```python
from build123d import *

# Parameters (mm, degrees)
SKETCH1_W           = 500
SKETCH1_H           = 775
BOSS_EXTRUDE1_DEPTH = 50
SKETCH2_R           = 8
CUT_EXTRUDE1_DEPTH  = 45
CUT_EXTRUDE2_START  = -45
SKETCH3_R           = 8
CUT_EXTRUDE2_DEPTH  = 45
SKETCH4_R           = 66.548277476
BOSS_EXTRUDE2_DEPTH = 60.75
FILLET1_R           = 60


with BuildPart() as part:
    # Sketch1 → Boss-Extrude1 (new body)
    with BuildSketch(Plane(origin=(0, 0, 0), x_dir=(1, 0, 0), z_dir=(0, 1, 0))):
        with Locations((250, 387.5)):
            Rectangle(SKETCH1_W, SKETCH1_H)
    extrude(amount=BOSS_EXTRUDE1_DEPTH)

    # Sketch2 → Cut-Extrude1 (cut)
    with BuildSketch(Plane(origin=(500, 0, 0), x_dir=(0, 0, -1), z_dir=(1, 0, 0))):
        with Locations((387.5, 25)):
            Circle(SKETCH2_R)
    extrude(amount=-CUT_EXTRUDE1_DEPTH, mode=Mode.SUBTRACT)

    # Sketch3 → Cut-Extrude2 (cut)
    with BuildSketch(Plane.ZY.offset(CUT_EXTRUDE2_START)):
        with Locations(Location((-387.5, 25, 0), (0, 0, 180))):
            Circle(SKETCH3_R)
    extrude(amount=CUT_EXTRUDE2_DEPTH, mode=Mode.SUBTRACT)

    # Sketch4 → Boss-Extrude2 (add)
    with BuildSketch(Plane(origin=(0, 0, 0), x_dir=(-1, 0, 0), z_dir=(0, -1, 0))):
        with Locations(Location((-250, 100, 0), (0, 0, 90))):
            Circle(SKETCH4_R)
    extrude(amount=BOSS_EXTRUDE2_DEPTH)

    # Fillet1
    fillet1_edges = [part.edges().sort_by_distance(p)[0] for p in [
        (250, -60.75, -33.451722524),
    ]]
    fillet(fillet1_edges, radius=FILLET1_R)


solid = part.part
```
Read the model definition and answer for the solid it produces. Units are mm, in the model's axes. A direction names the side the tool comes from. Coordinates: 2 decimals unless noted, no trailing zeros. Write each loop counter-clockwise with the first axis right and the second up, starting at its lowest first coordinate (ties: lowest second). Pieces come first, ordered by that corner, then holes. Notation, with made-up numbers: (-5, -30) - (45, -30) arc R25 cw to (45, -2) - close; hole circle Ø7 at (60.25, -17). An arc over 180 degrees is marked (long way). Answer as a JSON object with one key per item and string values. Group by question number.
1. A cutting plane is placed at B-B (x = 366.5). Determine the outline of the cut face in (y, z), plus the area to 4 significant figures.
2. The mould has two halves that part along Y. Classify faces 6 (the cylindrical face through (22.82, 22.6, -395.13)), 7 (the flat face through (247, 0, -393)), 8 (the flat face through (500, 14, -382)): +Y half, -Y half, draft (parallel to the pull), parting line (faces both ways), or undercut.
3. Which of the six approach directions +Z, -Z, +X, -X, +Y, -Y give full straight-line access (tool end or side, diameter ignored) to faces 1 (the flat face through (45, 25, -387)), 2 (the flat face through (247, 25, 0)), 3 (the cylindrical face through (477.82, 27.4, -395.13)), 4 (the cylindrical face through (294.976, -0.37, -50.951)), 5 (the flat face through (0, 14, -382))?
4. A cutting plane is placed at A-A (z = -387.5). Determine the outline of the cut face in (x, y), plus the area to 3 significant figures.
5. Each of these flat-tipped pins is pushed along its axis until it touches: P1, Ø5, axis at y = 27, z = -386, coming from the +X side; P2, Ø1.5, axis at x = 153.5, z = -663, coming from the -Y side; P3, Ø10, axis at x = 308.5, y = -26, coming from the +Z side. Where does it stop, or does it pass through?
6. Consider L1, parallel to Z at x = 33, y = 25; L2, parallel to Y at x = 18, z = -387; L3, parallel to Y at x = 466.5, z = -374. Determine where each line is inside the solid, lowest interval first. Write a range as [from, to].
Worked out:
{
 "1": {"outline": "(0, -775) - (50, -775) - (50, 0) - (0, 0) - close", "area": "38,750 mm²"},
 "2": {"face 6": "undercut", "face 7": "-Y half", "face 8": "draft"},
 "3": {"face 1": "-X", "face 2": "+Z, +X, -X, +Y, -Y", "face 3": "+X", "face 4": "-Y", "face 5": "+Z, -Z, -X, +Y, -Y"},
 "4": {"outline": "(0, 0) - (500, 0) - (500, 17) - (455, 17) - (455, 33) - (500, 33) - (500, 50) - (0, 50) - (0, 33) - (45, 33) - (45, 17) - (0, 17) - close", "area": "23,600 mm²"},
 "5": {"P1": "stops at x = 455", "P2": "stops at y = 0", "P3": "stops at z = -69.67"},
 "6": {"L1": "z = [-775, -395.5], [-379.5, 0]", "L2": "y = [0, 17.02], [32.98, 50]", "L3": "y = [0, 50]"}
}
